from build123d import *

# Parameters (mm, degrees)
SKETCH1_R           = 13.5
BOSS_EXTRUDE1_DEPTH = 5
SKETCH2_R           = 11.5
SKETCH2_R_2         = 10.75
BOSS_EXTRUDE2_DEPTH = 10
SKETCH3_R           = 6
BOSS_EXTRUDE3_DEPTH = 10


with BuildPart() as part:
    # Sketch1 → Boss-Extrude1 (new body)
    with BuildSketch(Plane.XY):
        Circle(SKETCH1_R)
    extrude(amount=BOSS_EXTRUDE1_DEPTH)

    # Sketch2 → Boss-Extrude2 (add)
    with BuildSketch(Plane.XY.offset(5)):
        Circle(SKETCH2_R)
        Circle(SKETCH2_R_2, mode=Mode.SUBTRACT)
    extrude(amount=BOSS_EXTRUDE2_DEPTH)

    # Sketch3 → Boss-Extrude3 (add)
    with BuildSketch(Plane.XY.offset(5)):
        Circle(SKETCH3_R)
    extrude(amount=BOSS_EXTRUDE3_DEPTH)


solid = part.part
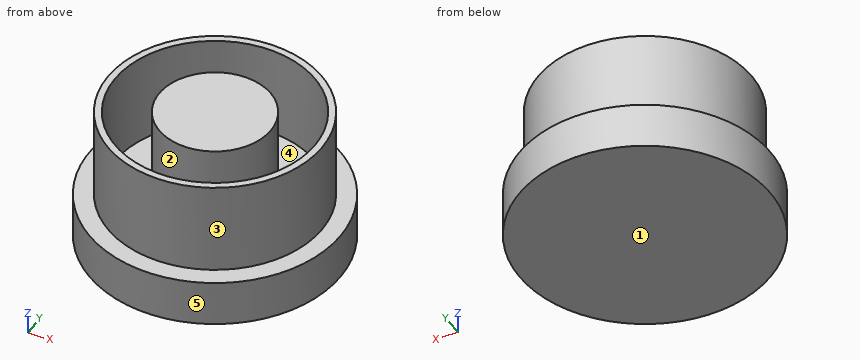
Could you check a few things on this model? Use its own coordinates, in mm. Face numbers are marked on the shaded views. A direction names the side the tool comes from. Give positions to 0.01 mm unless a question says otherwise; leave off trailing zeros. Loops run counter-clockwise (first coordinate to the right, second up) from the corner with the lowest first, then second, coordinate; pieces in that order, holes last. Notation, with made-up numbers: M 13,87 L 25,87 A6 cw 25,94 Z; hole C 26,-12 d6. An arc over 180 degrees is marked long. Answer as a JSON object with one key per item and string values.
Q1. If I drill on probe 1 along Y at (x, z) = (0, 9.75); probe 2 along Y at (x, z) = (-4.5, 10.5); probe 3 along X at (y, z) = (3.5, 14), over which ranges is the centre line in solid material (lowest first)? Write a range as [from, to].
Values found:
{"probe 1": "y = [-11.5, -10.75], [-6, 6], [10.75, 11.5]", "probe 2": "y = [-10.58, -9.76], [-3.97, 3.97], [9.76, 10.58]", "probe 3": "x = [-10.95, -10.16], [-4.87, 4.87], [10.16, 10.95]"}
Q2. Suppose I cut it at B-B, the plane y = 0. List the corners of the cut face in (x, z) for me, plus the area to 3 significant figures.
Values found:
{"outline": "M -13.5,0 L 13.5,0 L 13.5,5 L 11.5,5 L 11.5,15 L 10.75,15 L 10.75,5 L 6,5 L 6,15 L -6,15 L -6,5 L -10.75,5 L -10.75,15 L -11.5,15 L -11.5,5 L -13.5,5 Z", "area": "270 mm²"}
Q3. Suppose I cut it at A-A, the plane z = 7.5. List the corners of the cut face in (x, y) for me.
Values found:
{"outline": "C 0,0 d23; C 0,0 d12; hole C 0,0 d21.5"}
Q4. For P1, Ø8, axis at x = -10.5, z = 4.5, coming from the +Y side; P2, Ø1.5, axis at y = 9, z = 10.5, coming from the +X side; P3, Ø2, axis at y = -7.5, z = 13.5, coming from the +X side; P4, Ø12, axis at x = 4, y = -8.5, coming from the -Z side, each with a flat end and sliding along its axis, tell me the tip position at first contact or that it passes through.
Values found:
{"P1": "stops at y = 11.83", "P2": "stops at x = 8.01", "P3": "stops at x = 9.49", "P4": "stops at z = 0"}
Q5. If we mould it in two halves opening along Y, with no side actions, what happens to the marked faces 1, 2 and 3? For each: pulls with the +Y half, pulls with the -Y half, needs draft (parallel to the pull), parting line crosses it, or undercut.
Values found:
{"face 1": "needs draft", "face 2": "undercut", "face 3": "parting line crosses it"}
Q6. For the marked faces 4 and 5, which set-ups out of +Z, -Z, +X, -X, +Y, -Y let a thin tool reach every point of the face, with its end or its side?
Values found:
{"face 4": "+Z", "face 5": "+Z, -Z"}
Q7. Suppose I cut it at D-D, the plane y = 7.5. List the corners of the cut face in (x, z) for me, plus the area to 3 significant figures.
Values found:
{"outline": "M -11.22,0 L 11.22,0 L 11.22,5 L 8.72,5 L 8.72,15 L 7.7,15 L 7.7,5 L -7.7,5 L -7.7,15 L -8.72,15 L -8.72,5 L -11.22,5 Z", "area": "133 mm²"}
